Geometry check sheet. Reference: the model listing, model coordinates, mm. Face numbers are marked on the shaded views. A direction names the side the tool comes from. Coordinates: 2 decimals unless noted, no trailing zeros. Write each loop counter-clockwise with the first axis right and the second up, starting at its lowest first coordinate (ties: lowest second). Pieces come first, ordered by that corner, then holes.
from build123d import *

# Parameters (mm, degrees)
SKETCH2_W           = 100
SKETCH2_H           = 300
BOSS_EXTRUDE1_DEPTH = 75
CUT_EXTRUDE1_REACH  = 422.463
CUT_EXTRUDE1_START  = 150
SKETCH3_W           = 100
SKETCH3_H           = 110
SKETCH4_R           = 10
BOSS_EXTRUDE2_DEPTH = 110
SKETCH5_R           = 12.5
BOSS_EXTRUDE3_DEPTH = 100
FILLET1_RADIUS      = 50
FILLET1_LENGTH      = 110
FILLET2_R           = 10
FILLET3_R           = 10


with BuildPart() as part:
    # Sketch2 → Boss-Extrude1 (new, symmetric)
    with BuildSketch(Plane.XY):
        Rectangle(SKETCH2_W, SKETCH2_H)
        with BuildLine():
            ThreePointArc((-50, 205), (0, 255), (50, 205))
            Line((50, 205), (50, 150))
            Line((50, 150), (-50, 150))
            Line((-50, 150), (-50, 205))
        make_face()
    extrude(amount=BOSS_EXTRUDE1_DEPTH, both=True)

    # Sketch3 → Cut-Extrude1 (cut, up to next)
    with BuildSketch(Plane(origin=(0, 0, 0), x_dir=(1, 0, 0), z_dir=(0, 1, 0)).offset(CUT_EXTRUDE1_START), mode=Mode.PRIVATE) as cut_extrude1_sk1:
        Rectangle(SKETCH3_W, SKETCH3_H)
    cut_extrude1_tool1 = extrude(cut_extrude1_sk1.sketch, amount=CUT_EXTRUDE1_REACH, mode=Mode.PRIVATE) & part.part
    add(cut_extrude1_tool1.solids().sort_by_distance((0, 150, 0))[0], mode=Mode.SUBTRACT)

    # Sketch4 → Boss-Extrude2 (add)
    with BuildSketch(Plane.XY.offset(-55)):
        with Locations(Location((0, 205, 0), (0, 0, 180))):
            Circle(SKETCH4_R)
    extrude(amount=BOSS_EXTRUDE2_DEPTH)

    # Sketch5 → Boss-Extrude3 (add)
    with BuildSketch(Plane.XZ.offset(150)):
        with Locations(Location((0, 0, 0), (0, 0, 90))):
            Circle(SKETCH5_R)
    extrude(amount=BOSS_EXTRUDE3_DEPTH)

    # Fillet1: full round fillet: the end face becomes a half cylinder, R = half its width
    fillet1_face = Plane((0, 150, 0), x_dir=(0, 0, -1), z_dir=(0, 1, 0))  # on the end face: x along it, z out of the body
    fillet1_slab = fillet1_face.offset(-FILLET1_RADIUS / 2) * Box(FILLET1_LENGTH, 2 * FILLET1_RADIUS, FILLET1_RADIUS, mode=Mode.PRIVATE)  # the body's end, R deep
    fillet1_round = Plane((0, 100, 0), x_dir=(0, 1, 0), z_dir=(0, 0, -1)) * Cylinder(FILLET1_RADIUS, FILLET1_LENGTH, mode=Mode.PRIVATE)  # its axis R under the face
    add(fillet1_slab - fillet1_round, mode=Mode.SUBTRACT)

    # Fillet2
    fillet2_edges = [part.edges().sort_by_distance(p)[0] for p in [
        (0, 255, 75),
        (-50, 27.5, 75),
        (0, -150, 75),
        (50, 27.5, 75),
        (0, -150, -75),
        (-50, 27.5, -75),
        (0, 255, -75),
        (50, 27.5, -75),
        (50, -150, 0),
        (-50, -150, 0),
    ]]
    fillet(fillet2_edges, radius=FILLET2_R)

    # Fillet3
    fillet3_edges = [part.edges().sort_by_distance(p)[0] for p in [
        (50, 152.5, 55),
        (0, 255, 55),
        (50, 152.5, -55),
        (0, 255, -55),
        (-50, 152.5, 55),
        (-50, 152.5, -55),
    ]]
    fillet(fillet3_edges, radius=FILLET3_R - 0.0001)  # a hair under: the kernel refuses the full size


solid = part.part
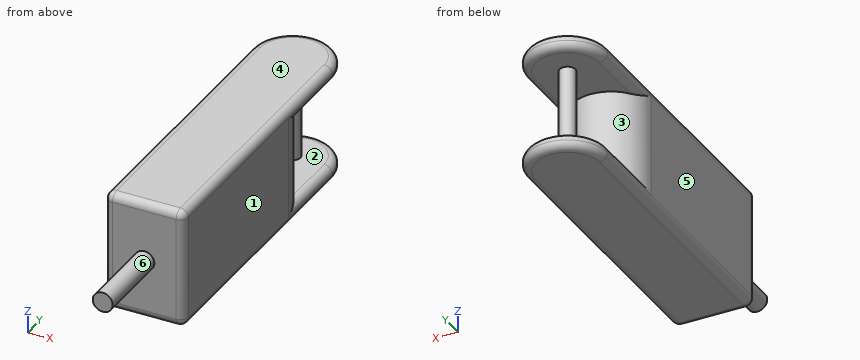
1. Access from +Z, -Z, +X, -X, +Y, -Y to the whole of each face (thin tool, end or side, straight path). Record for the marked faces 1 and 2.
Computed values:
face 1: +Z, -Z, +X, +Y, -Y
face 2: none
2. Sectioned sample at A-A, the plane z = 0. Record the boundary of the cut face in (x, y), and give its area (3 significant figures).
Computed values:
outline: (-50, -140) arc R10 ccw to (-40, -150) - (-12.5, -150) - (-12.5, -250) - (12.5, -250) - (12.5, -150) - (40, -150) arc R10 ccw to (50, -140) - (50, 100) arc R50 ccw to (-50, 100) - close; circle Ø20 at (0, 205)
area: 31,700 mm2
3. Sectioned sample at C-C, the plane z = -21. Record the boundary of the cut face in (x, y), and give its area (3 significant figures).
Computed values:
outline: (-50, -140) arc R10 ccw to (-40, -150) - (40, -150) arc R10 ccw to (50, -140) - (50, 100) arc R50 ccw to (-50, 100) - close; circle Ø20 at (0, 205)
area: 29,200 mm2
4. Draft check along Z on the marked faces 3, 4, 5 and 6. Enter one of: released by +Z, released by -Z, zero draft, split by the parting line, or undercut.
Computed values:
face 3: undercut
face 4: released by +Z
face 5: zero draft
face 6: split by the parting line
5. Gauge pin test, flat ends, axial feed: pin 1 Ø4 at (x, z) = (21.5, -10) entering from -Y; pin 2 Ø10 at (y, z) = (120, -51) entering from -X; pin 3 Ø10 at (x, z) = (-32.5, -42) entering from +Y. Record the tip position at first contact, or that the pin passes through.
Computed values:
pin 1: stops at y = -150
pin 2: stops at x = -47.7
pin 3: stops at y = 141.76
6. Thickness scan on line 1 along Y through (x, z) = (-8.5, 54); line 2 along Y through (x, z) = (-33.5, 62.5); line 3 along X through (y, z) = (181, -56). Record the ranges inside material, lowest first.
Computed values:
line 1: y = -150 to 149.27, 199.73 to 210.27
line 2: y = -150 to 241.69
line 3: x = -44.36 to 44.36
